For this review, take the finished solid that the model builds, in its own axes (mm). Face numbers are marked on the shaded views. Coordinates: 2 decimals unless noted, no trailing zeros. Order: outer loops, then holes, each group sorted by start corner. A loop starts at its lowest first (then second) coordinate and runs counter-clockwise, first axis right, second up.
from build123d import *

# Parameters (mm, degrees)
CROQUIS2_R            = 9.525
CORTAR_EXTRUIR1_DEPTH = 40


with BuildPart() as part:
    # Croquis1 → Revolución1 (revolve)
    with BuildSketch(Plane.XY, mode=Mode.PRIVATE) as revoluci_n1_sk:
        with BuildLine():
            Line((0, 0), (0, 14.525))
            Line((0, 14.525), (-38.1, 14.525))
            Line((-38.1, 14.525), (-38.1, 9.525))
            ThreePointArc((-38.1, 9.525), (-31.364807909, 6.735192091), (-28.575, 0))
            Line((-28.575, 0), (0, 0))
        make_face()
        with BuildLine():
            Line((0, -14.525), (0, 0))
            Line((0, 0), (-28.575, 0))
            ThreePointArc((-28.575, 0), (-31.364807909, -6.735192091), (-38.1, -9.525))
            Line((-38.1, -9.525), (-38.1, -14.525))
            Line((-38.1, -14.525), (0, -14.525))
        make_face()
    revolve(revoluci_n1_sk.sketch.rotate(Axis((0, 62.433588071, 0), (0, -1, 0)), 270), axis=Axis((0, 62.433588071, 0), (0, -1, 0)))

    # Croquis2 → Cortar-Extruir1 (cut)
    with BuildSketch(Plane(origin=(0, 14.525, 0), x_dir=(1, 0, 0), z_dir=(0, 1, 0))):
        with Locations(Location((0, 0, 0), (0, 0, 270))):
            Circle(CROQUIS2_R)
    extrude(amount=-CORTAR_EXTRUIR1_DEPTH, mode=Mode.SUBTRACT)


solid = part.part
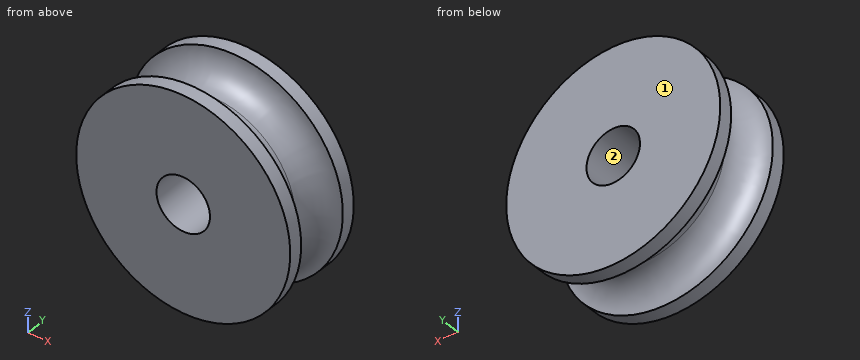
1. The part is to be moulded in two halves that separate along Z. For the marked faces 1 and 2, say which applies: +Z half, -Z half, draft (parallel to the pull), parting line (faces both ways), or undercut.
Answer below:
face 1: draft
face 2: undercut
2. To check wall thickness, follow L1, parallel to X at y = -2.5, z = -2; L2, parallel to Y at x = -31, z = 20.5 (3 decimals); L3, parallel to Y at x = 32, z = -17 (3 decimals). State the ranges of each line that lie inside material, in increasing order.
Answer below:
L1: x = -28.84 to -9.31, 9.31 to 28.84
L2: y = -14.525 to -9.479, 9.479 to 14.525
L3: y = -14.525 to -9.341, 9.341 to 14.525
3. Clearance check with flat-ended pins moving along their axes: pin 1 Ø1.5 at (y, z) = (-4, 23.5) entering from +X; pin 2 Ø4 at (x, y) = (-27, 2) entering from -Z; pin 3 Ø10 at (x, y) = (-12, 7) entering from +Z. State where each tip first meets the part, or that it passes through.
Answer below:
pin 1: stops at x = 18.88
pin 2: stops at z = -14.41
pin 3: stops at z = 37.32
4. Take a section at B-B, the plane y = -7.5. Give the boundary of the cut face in (x, z) (3 decimals), plus the area to 3 significant figures.
Answer below:
outline: circle Ø64.457 at (0, 0); hole circle Ø19.05 at (0, 0)
area: 2,980 mm2
5. Take a section at A-A, the plane y = 10.5. Give the boundary of the cut face in (x, z) (3 decimals).
Answer below:
outline: circle Ø76.2 at (0, 0); hole circle Ø19.05 at (0, 0)
